Autodesk Inventor part; units mm, degrees
ref_plane "YZ Plane" through (0, 0, 0) normal (1, 0, 0) x (0, 1, 0)
ref_plane "XZ Plane" through (0, 0, 0) normal (0, 1, 0) x (-1, 0, 0)
ref_plane "XY Plane" through (0, 0, 0) normal (0, 0, 1) x (1, 0, 0)
sketch "Sketch1" plane through (0, 0, 0) normal (0, 1, 0) x (-1, 0, 0)
  circle A0 centre (0, 0) radius 40
  circle A1 centre (0, 0) radius 50
  dimension "d0" = 80
  dimension "d1" = 100
extrude "Extrusion1" add sketch "Sketch1" along normal blind 2
sketch "Sketch2" plane through (0, 0, 0) normal (0, 1, 0) x (-1, 0, 0)
  line L0 (0, 0) -> (-39.598, 39.598) construction
  circle A0 centre (0, 0) radius 50 construction
  line L1 (-31.6426, 38.7137) -> (-36.0624, 43.1335)
  line L2 (-36.0624, 43.1335) -> (-39.598, 39.598)
  line L3 (70, 0) -> (-70, 0) construction
  line L4 (-38.7137, 31.6426) -> (-43.1335, 36.0624)
  line L5 (-43.1335, 36.0624) -> (-39.598, 39.598)
  arc A1 (-31.6426, 38.7137) -> (-38.7137, 31.6426) centre (0, 0) ccw
  dimension "d4" = 56
  dimension "d6" = 5
  dimension "d7" = 45
extrude "Extrusion2" add sketch "Sketch2" along normal blind 2
fillet "Fillet1" radius 2 2 edges at (43.1335, 1, 36.0624) (36.0624, 1, 43.1335)
sketch "Sketch3" plane through (0, 0, 0) normal (0, -1, 0) x (1, 0, 0)
  line L0 (0, 0) -> (39.598, 39.598) construction
  line L1 (37.4767, 41.7193) -> (41.7193, 37.4767) construction
  point P0 (35.3553, 35.3553)
  dimension "d11" = 50
hole "Hole1" at (35.3553, 0, 35.3553) direction (0, 1, 0) diameter 3.4 end through all
pattern_circular "Circular Pattern1" count 4 over 360 about axis through (0, -10, 0) along (0, 1, 0) of "Hole1", "Fillet1", "Extrusion2"
properties part number "Succ_Plate"
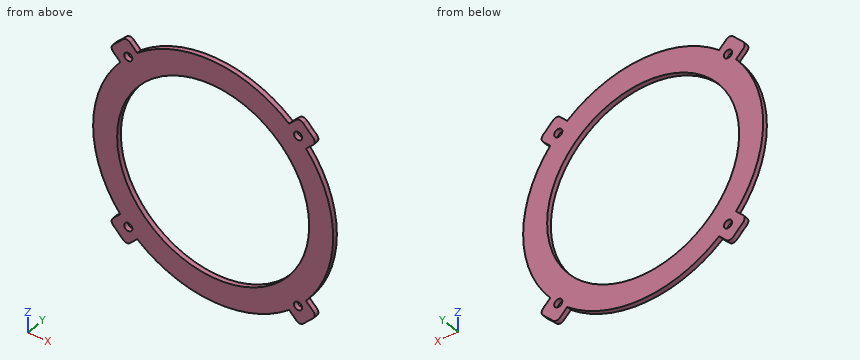
CAD build for the part. Positions are in the model's coordinates, mm. Coordinates: 2 decimals unless noted, no trailing zeros. Order: outer loops, then holes, each group sorted by start corner. A loop starts at its lowest first (then second) coordinate and runs counter-clockwise, first axis right, second up.
(1) Saw through at C-C, the plane y = 0.45. Count the separate pieces of the cut face and the enclosed holes in it, and give its area (3 significant figures).
Solution:
separate pieces: 1
enclosed holes: 5
area: 3,030 mm2
(2) Pin check, flat tips, straight feed: pin 1 Ø1 at (y, z) = (1.5, 30.5) entering from +X; pin 2 Ø2.5 at (x, z) = (35.36, -35.36) entering from -Y. Stop position of each tip, or through.
Solution:
pin 1: stops at x = 40
pin 2: passes through
(3) Drill centre lines: L1, parallel to Z at x = -34.5, y = 0.4; L2, parallel to X at y = 0.25, z = 0.5; L3, parallel to Z at x = -1, y = 0.6. Where is each one in solid material? Low to high.
Solution:
L1: z = -41.57 to -36.82, -33.89 to -20.24, 20.24 to 33.89, 36.82 to 41.57
L2: x = -50 to -40, 40 to 50
L3: z = -49.99 to -39.99, 39.99 to 49.99
(4) Saw through at A-A, the plane z = 0. Write the cut outline in (x, y), and give its area (3 significant figures).
Solution:
outline: (-50, 0) - (-40, 0) - (-40, 2) - (-50, 2) - close; (40, 0) - (50, 0) - (50, 2) - (40, 2) - close
area: 40.0 mm2
(5) Saw through at B-B, the plane x = 0. Write the cut outline in (y, z), and give its area (3 significant figures).
Solution:
outline: (0, -50) - (2, -50) - (2, -40) - (0, -40) - close; (0, 40) - (2, 40) - (2, 50) - (0, 50) - close
area: 40.0 mm2
